from build123d import *

# Parameters (mm, degrees)
F1_DEPTH = 50.8
F2_W     = 50.8
F2_H     = 101.6
F3_DEPTH = 76.2
F4_SIZE  = 50.8


with BuildPart() as f1:
    # F0 (on Top) → F1 (new body)
    with BuildSketch(Plane.XY):
        Polygon((101.6, 16.512535), (-101.6, 16.512535), (-101.6, -85.087465), (101.6, -85.087465), (101.6, -59.687465), (0, -59.687465), (0, -8.887465), (101.6, -8.887465), align=None)
    extrude(amount=F1_DEPTH)

    # F2 (on face) → F3 (join)
    with BuildSketch(Plane.XY.offset(50.8)):
        with Locations((-76.2, -34.287465)):
            Rectangle(F2_W, F2_H)
    extrude(amount=F3_DEPTH)

    # F4
    f4_edges = [f1.edges().sort_by_distance(p)[0] for p in [
        (-76.2, -85.087465, 127),
    ]]
    chamfer(f4_edges, length=F4_SIZE)


solid = f1.part
The listing builds one solid part. Answer for the finished solid, in the listing's coordinates (mm). A direction names the side the tool comes from. Give positions to 0.01 mm unless a question says otherwise; leave off trailing zeros. Write each loop counter-clockwise with the first axis right and the second up, starting at its lowest first coordinate (ties: lowest second). Pieces come first, ordered by that corner, then holes. Notation, with made-up numbers: (61, -29) - (91, -29) arc R29 ccw to (91, -6) - close; hole circle Ø11 at (85, 9). An arc over 180 degrees is marked (long way). One line per question, with ' | ' between items. Start each with the question number.
1. Determine the mould class of faces 1 (the face through (0, -35, 25)), 2 (the face through (-1, -85.087, 29)), 3 (the face through (101.6, -73, 25)), 4 (the face through (50, -8.887, 25)) for opening direction Y: +Y half, -Y half, draft (parallel to the pull), parting line (faces both ways), or undercut.
2. Section B-B, the plane z = 43 is taken. Determine the outline of the cut face in (x, y), then the cut area to 3 significant figures.
3. Straight lines are drawn through the part: line 1 (Y direction, x = 10, z = 35); line 2 (X direction, y = -17, z = 30.5); line 3 (Z direction, x = -29, y = -43). For each, find the intervals that lie inside material, in ascending order.
4. For faces 5 (the face through (-10, -34, 50.8)), 6 (the face through (-24, 16.513, 34)), 7 (the face through (52, -59.687, 25)), determine the directions among +Z, -Z, +X, -X, +Y, -Y from which every point of the face is accessible in a straight line to the end or side of a thin tool.
5. Given P1, Ø1, axis at x = -71, z = 81, coming from the -Y side; P2, Ø5, axis at x = -25.5, y = -66, coming from the +Z side; P3, Ø5, axis at y = -61, z = 85, coming from the +X side, each flat-ended and moving along its own axis, determine where each tip first touches the part or whether it passes through.
6. Section C-C, the plane y = -25.5 is taken. Determine the outline of the cut face in (x, z), then the cut area to 3 significant figures.
7. Section D-D, the plane x = -76.5 is taken. Determine the outline of the cut face in (y, z).
8. Section A-A, the plane x = 24.5 is taken. Determine the outline of the cut face in (y, z).
Result:
1) face 1: undercut | face 2: -Y half | face 3: draft | face 4: undercut
2) outline: (-101.6, -85.09) - (101.6, -85.09) - (101.6, -59.69) - (0, -59.69) - (0, -8.89) - (101.6, -8.89) - (101.6, 16.51) - (-101.6, 16.51) - close | area: 15,500 mm2
3) line 1: y = -85.09 to -59.69, -8.89 to 16.51 | line 2: x = -101.6 to 0 | line 3: z = 0 to 50.8
4) face 5: +Z, +X, +Y, -Y | face 6: +Z, -Z, +X, -X, +Y | face 7: +Z, -Z, +X
5) P1: stops at y = -80.79 | P2: stops at z = 50.8 | P3: stops at x = -50.8
6) outline: (-101.6, 0) - (0, 0) - (0, 50.8) - (-50.8, 50.8) - (-50.8, 127) - (-101.6, 127) - close | area: 9,030 mm2
7) outline: (-85.09, 0) - (16.51, 0) - (16.51, 127) - (-34.29, 127) - (-85.09, 76.2) - close
8) outline: (-85.09, 0) - (-59.69, 0) - (-59.69, 50.8) - (-85.09, 50.8) - close; (-8.89, 0) - (16.51, 0) - (16.51, 50.8) - (-8.89, 50.8) - close
